CAD build for the part. Positions are in the model's coordinates, mm. Give positions to 0.01 mm unless a question says otherwise; leave off trailing zeros. Write each loop counter-clockwise with the first axis right and the second up, starting at its lowest first coordinate (ties: lowest second). Pieces come first, ordered by that corner, then holes. Notation, with made-up numbers: (30.25, 71.25) -> (47.25, 71.25) arc R29 ccw to (47.25, 92.25) -> close; hole circle Ø10 at (3.5, 13). An arc over 180 degrees is marked (long way). Answer in a Markdown table with one row per item. Add a question column.
```python
from build123d import *

# Parameters (mm, degrees)
F0_R     = 127
F1_DEPTH = 63.5


with BuildPart() as f1:
    # F0 (on Front) → F1 (new body, symmetric)
    with BuildSketch(Plane.XZ):
        with BuildLine():
            Line((-203.2, 0), (-203.2, -1143))
            Line((-203.2, -1143), (203.2, -1143))
            Line((203.2, -1143), (203.2, 0))
            ThreePointArc((203.2, 0), (0, 203.2), (-203.2, 0))
        make_face()
        Circle(F0_R, mode=Mode.SUBTRACT)
    extrude(amount=F1_DEPTH, both=True)


solid = f1.part
```
Item 1: Slice it at A-A, the plane x = 0. List the corners of the cut face in (y, z).
Item 2: Probe L1, parallel to Z at x = -6, y = -56; L2, parallel to Z at x = 0, y = 30; L3, parallel to X at y = 43.5, z = -48.5. List the from-to ranges inside material, lowest first. Write a range as from..to.
Item 3: Mould opens along X. For faces 1 (the face through (203.2, -1, -580)), 2 (the face through (4.47, -0.89, 203.15)), 3 (the face through (-27.53, 0.89, -123.98)), 4 (the face through (-3, -63.5, -460)) say: released by +X, released by -X, zero draft, split by the parting line, or undercut.
Item 4: Slice it at C-C, the plane y = 15. List the corners of the cut face in (x, z), then the cut area to 3 significant figures.
Item 5: Slice it at B-B, the plane z = 91. List the corners of the cut face in (x, y).
Item 6: Slice it at D-D, the plane x = 162. List the corners of the cut face in (y, z).
Answer key:
| question | item | result |
|---|---|---|
| 1 | outline | (-63.5, -1143) -> (63.5, -1143) -> (63.5, -127) -> (-63.5, -127) -> close; (-63.5, 127) -> (63.5, 127) -> (63.5, 203.2) -> (-63.5, 203.2) -> close |
| 2 | L1 | z = -1143..-126.86, 126.86..203.11 |
| 2 | L2 | z = -1143..-127, 127..203.2 |
| 2 | L3 | x = -203.2..-117.37, 117.37..203.2 |
| 3 | face 1 | released by +X |
| 3 | face 2 | split by the parting line |
| 3 | face 3 | undercut |
| 3 | face 4 | zero draft |
| 4 | outline | (-203.2, -1143) -> (203.2, -1143) -> (203.2, 0) arc R203.2 ccw to (-203.2, 0) -> close; hole circle Ø254 at (0, 0) |
| 4 | area | 479,000 mm² |
| 5 | outline | (-181.68, -63.5) -> (-88.59, -63.5) -> (-88.59, 63.5) -> (-181.68, 63.5) -> close; (88.59, -63.5) -> (181.68, -63.5) -> (181.68, 63.5) -> (88.59, 63.5) -> close |
| 6 | outline | (-63.5, -1143) -> (63.5, -1143) -> (63.5, 122.66) -> (-63.5, 122.66) -> close |
